Geometry: final body of the model. Coordinates: model frame, mm. Face numbers are marked on the shaded views. A direction names the side the tool comes from. Give positions to 0.01 mm unless a question says otherwise; leave off trailing zeros. Write each loop counter-clockwise with the first axis right and the second up, starting at its lowest first coordinate (ties: lowest second). Pieces come first, ordered by that corner, then holes. Notation, with made-up numbers: M 27,0 L 81,0 A17 cw 81,11 Z; hole C -14.5,43 d2. An arc over 180 degrees is marked long. Use a Markdown table: item, result. Add a question column.
1) Pin query (flat end, axial travel): pin 1 (0.8 mm diameter, centred on y = -11.5, z = 1.5, fed in from +X); pin 2 (1.5 mm diameter, centred on y = -16, z = 1.5, fed in from -X); pin 3 (0.5 mm diameter, centred on x = -4.5, z = 2, fed in from +Y). Return the tip coordinate at first contact, or that it passes through.
2) Line query: line 1 (Y direction, x = 0, z = 1.35); line 2 (Y direction, x = -1.25, z = 1.4); line 3 (X direction, y = -14.25, z = 1.75). Output: solid intervals per line, ascending.
3) Section D-D on x = -11. Return the cut outline in (y, z).
4) Set-up query: the marked faces 1 and 2. Return all of +Z, -Z, +X, -X, +Y, -Y with unobstructed straight access to the full face (end or side cutting, diameter ignored); none if empty.
5) Section A-A on x = 0.25. Return the cut outline in (y, z).
6) Section C-C on z = 1.8. State how many separate pieces and enclosed holes the cut face has, then the cut area to 3 significant figures.
7) Section B-B on y = -18. Return the cut outline in (x, z), then the cut area to 3 significant figures.
8) Draft query along Y for the marked faces 3, 4 and 5. Return one class per face: +Y half, -Y half, draft (parallel to the pull), parting line (faces both ways), or undercut.
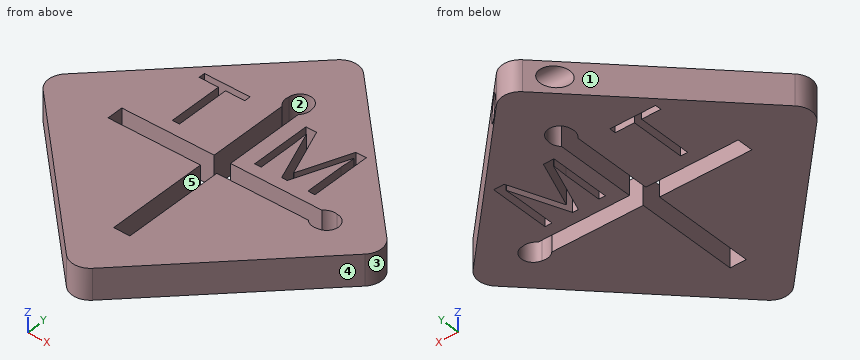
```python
from build123d import *

# Parameters (mm, degrees)
F1_DEPTH = 2.5
F2_R     = 0.85
F3_DEPTH = 12.5


with BuildPart() as f1:
    # F0 (on Top) → F1 (new body)
    with BuildSketch(Plane.XY):
        with BuildLine():
            Line((13.081475452, -13.081475452), (1.0606601718, -1.0606601718))
            ThreePointArc((1.0606601718, -1.0606601718), (0, -0.6213203436), (-1.0606601718, -1.0606601718))
            Line((-1.0606601718, -1.0606601718), (-13.081475452, -13.081475452))
            ThreePointArc((-13.081475452, -13.081475452), (-13.5208152802, -14.1421356237), (-13.081475452, -15.2027957955))
            Line((-13.081475452, -15.2027957955), (-1.0606601718, -27.2236110757))
            ThreePointArc((-1.0606601718, -27.2236110757), (0, -27.6629509039), (1.0606601718, -27.2236110757))
            Line((1.0606601718, -27.2236110757), (13.081475452, -15.2027957955))
            ThreePointArc((13.081475452, -15.2027957955), (13.5208152802, -14.1421356237), (13.081475452, -13.081475452))
        make_face()
        Polygon((-4.3332411349, -7.9814997978), (-4.3332411349, -12.4270293117), (-4.9094130099, -12.4270293117), (-4.9094130099, -7.9814997978), (-6.479508496, -7.9814997978), (-6.479508496, -7.46934702), (-2.7631456488, -7.46934702), (-2.7631456488, -7.9814997978), align=None, mode=Mode.SUBTRACT)
        with BuildLine():
            Line((-8.1334756687, -14.8039748892), (-8.1334756687, -13.4802963582))
            Line((-8.1334756687, -13.4802963582), (-0.6236797201, -13.4802963582))
            Line((-0.6236797201, -13.4802963582), (-0.6236797201, -6.9198086858))
            ThreePointArc((-0.6236797201, -6.9198086858), (-0.9032194318, -6.4583786209), (-0.9135835525, -5.9189782686))
            ThreePointArc((-0.9135835525, -5.9189782686), (0.0168397474, -5.0141534426), (0.9868078824, -5.876451129))
            ThreePointArc((0.9868078824, -5.876451129), (0.9900106564, -6.4384308628), (0.6999988109, -6.9198086858))
            Line((0.6999988109, -6.9198086858), (0.6999988109, -13.4802963582))
            Line((0.6999988109, -13.4802963582), (8.1334756687, -13.4802963582))
            ThreePointArc((8.1334756687, -13.4802963582), (8.5949057336, -13.2007566465), (9.134306086, -13.1903925258))
            ThreePointArc((9.134306086, -13.1903925258), (10.0391309119, -14.1208158258), (9.1768332255, -15.0907839607))
            ThreePointArc((9.1768332255, -15.0907839607), (8.6148534917, -15.0939867347), (8.1334756687, -14.8039748892))
            Line((8.1334756687, -14.8039748892), (0.6999988109, -14.8039748892))
            Line((0.6999988109, -14.8039748892), (0.6999988109, -23.1867600232))
            Line((0.6999988109, -23.1867600232), (-0.6236797201, -23.1867600232))
            Line((-0.6236797201, -23.1867600232), (-0.6236797201, -14.8039748892))
            Line((-0.6236797201, -14.8039748892), (-8.1334756687, -14.8039748892))
        make_face(mode=Mode.SUBTRACT)
        with BuildLine():
            Line((4.530735705, -12.5424201787), (4.0663259828, -12.5424201787))
            Line((4.0663259828, -12.5424201787), (2.3844683439, -8.1478889287))
            Line((2.3844683439, -8.1478889287), (2.3573416078, -8.1478889287))
            add(Edge.make_bspline(
                [(2.3573416078, -8.1478889287), (2.4050846634, -8.6698073314), (2.4050846634, -9.3892083731)],
                knots=[0, 0, 0, 1, 1, 1], degree=2))
            Line((2.4050846634, -9.3892083731), (2.4050846634, -12.5424201787))
            Line((2.4050846634, -12.5424201787), (1.8723155662, -12.5424201787))
            Line((1.8723155662, -12.5424201787), (1.8723155662, -7.584737887))
            Line((1.8723155662, -7.584737887), (2.7403711217, -7.584737887))
            Line((2.7403711217, -7.584737887), (4.3104666078, -11.6743646231))
            Line((4.3104666078, -11.6743646231), (4.3375933439, -11.6743646231))
            Line((4.3375933439, -11.6743646231), (5.9207096634, -7.584737887))
            Line((5.9207096634, -7.584737887), (6.7822548023, -7.584737887))
            Line((6.7822548023, -7.584737887), (6.7822548023, -12.5424201787))
            Line((6.7822548023, -12.5424201787), (6.2060829273, -12.5424201787))
            Line((6.2060829273, -12.5424201787), (6.2060829273, -9.3479757342))
            add(Edge.make_bspline(
                [(6.2060829273, -9.3479757342), (6.2060829273, -8.7989305953), (6.2538259828, -8.1543993453)],
                knots=[0, 0, 0, 1, 1, 1], degree=2))
            Line((6.2538259828, -8.1543993453), (6.2266992467, -8.1543993453))
            Line((6.2266992467, -8.1543993453), (4.530735705, -12.5424201787))
        make_face(mode=Mode.SUBTRACT)
    extrude(amount=F1_DEPTH)

    # F2 (on Right) → F3 (cut, symmetric)
    with BuildSketch(Plane.YZ):
        with Locations((-2.4908210296, 1.292226194)):
            Circle(F2_R)
    extrude(amount=F3_DEPTH, both=True, mode=Mode.SUBTRACT)


solid = f1.part
```
Found:
| question | item | result |
|---|---|---|
| 1 | pin 1 | x = 11.9 |
| 1 | pin 2 | x = -13.03 |
| 1 | pin 3 | y = -4.25 |
| 2 | line 1 | -27.66 to -23.19, -5.01 to -3.34, -1.64 to -0.62 |
| 2 | line 2 | -27.03 to -14.8, -13.48 to -3.33, -1.65 to -1.25 |
| 2 | line 3 | -13.52 to -8.13, 10.03 to 13.52 |
| 3 | outline | M -17.28,0 L -11,0 L -11,2.5 L -17.28,2.5 Z |
| 4 | face 1 | +Z, -Z, -X, +Y |
| 4 | face 2 | +Z, -Z |
| 5 | outline | M -27.64,0 L -23.19,0 L -23.19,2.5 L -27.64,2.5 Z; M -5.04,0 L -0.64,0 L -0.64,2.5 L -5.04,2.5 Z; hole C -2.49,1.29 d1.7 |
| 6 | separate pieces | 2 |
| 6 | enclosed holes | 3 |
| 6 | area | 329 mm² |
| 7 | outline | M -10.28,0 L -0.62,0 L -0.62,2.5 L -10.28,2.5 Z; M 0.7,0 L 10.28,0 L 10.28,2.5 L 0.7,2.5 Z |
| 7 | area | 48.1 mm² |
| 8 | face 3 | parting line |
| 8 | face 4 | -Y half |
| 8 | face 5 | undercut |
